Autodesk Inventor part; units mm, degrees
ref_plane "YZ Plane" through (0, 0, 0) normal (1, 0, 0) x (0, 1, 0)
ref_plane "XZ Plane" through (0, 0, 0) normal (0, 1, 0) x (-1, 0, 0)
ref_plane "XY Plane" through (0, 0, 0) normal (0, 0, 1) x (1, 0, 0)
sketch "Boceto1" plane through (0, 0, 0) normal (1, 0, 0) x (0, 1, 0)
  line L0 (0, 0) -> (45, 0)
  line L1 (45, 0) -> (45, -18)
  line L2 (45, -18) -> (0, -18)
  line L3 (0, -18) -> (0, 0)
  dimension "d2" = 45
  dimension "d3" = 18
extrude "Extrusión1" add sketch "Boceto1" along normal blind 1
chamfer "Chaflán1" distance 1 angle 45 1 edges at (1, 0, -9)
fillet "Empalme1" radius 8 2 edges at (0.5, 45, -18) (0.5, 45, 0)
sketch "Boceto2" plane through (1, 0, 0) normal (1, 0, 0) x (0, 0, -1)
  point P0 (6.124, 36.1455)
hole "Agujero1" at (1, 36.1455, -6.124) direction (-1, 0, 0) diameter 3.4 end through all
properties part number "platina_3"
Verification items for the finished model (mm, model axes). Coordinates: 2 decimals unless noted, no trailing zeros. Order: outer loops, then holes, each group sorted by start corner. A loop starts at its lowest first (then second) coordinate and runs counter-clockwise, first axis right, second up. Notation, with made-up numbers: M 16,30 L 27,30 A16 cw 27,36 Z; hole C 88,40.5 d6. An arc over 180 degrees is marked long. Return JSON: item names as keys, results as strings.
1) Gauge pin test, flat end, axial feed: pin 1 (8 mm diameter, centred on y = 32, z = -4.5, fed in from -X). Record the tip position at first contact, or that the pin passes through.
Answer list:
{"pin 1": "x = 0"}
2) Cross-section at A-A, the plane x = 0.4. Record the boundary of the cut face in (y, z), and give its area (3 significant figures).
Answer list:
{"outline": "M 0.4,-18 L 37,-18 A8 ccw 45,-10 L 45,-8 A8 ccw 37,0 L 0.4,0 Z; hole C 36.15,-6.12 d3.4", "area": "766 mm2"}
3) Thickness scan on L1, parallel to Y at x = 0.85, z = -1.75; L2, parallel to Y at x = 0.2, z = -12; L3, parallel to Y at x = 0.3, z = -5.75. Record the ranges inside material, lowest first. Write a range as [from, to].
Answer list:
{"L1": "[0.85, 41.99]", "L2": "[0.2, 44.75]", "L3": "[0.3, 34.49], [37.8, 44.68]"}
4) Release check for a two-part mould opening along Y. For faces 1 (the flat face through (0.5, 0.5, -8.9)), 2 (the cylindrical face through (0.493, 37.805, -5.755)), 3 (the flat face through (1, 23, -9)) record: +Y half, -Y half, draft (parallel to the pull), parting line (faces both ways), or undercut.
Answer list:
{"face 1": "-Y half", "face 2": "undercut", "face 3": "draft"}
